Geometry: final body of the model. Coordinates: model frame, mm. A direction names the side the tool comes from. Give positions to 0.01 mm unless a question says otherwise; leave off trailing zeros. Write each loop counter-clockwise with the first axis right and the second up, starting at its lowest first coordinate (ties: lowest second). Pieces come first, ordered by that corner, then holes.
from build123d import *

# Parameters (mm, degrees)
REVOLUTION007_ANGLE     = 180
SKETCH064_W             = 14
SKETCH064_H             = 6
PAD026_DEPTH            = 10
SKETCH063_R             = 1.7
POCKET007_DEPTH         = 38.901
POCKET008_DEPTH         = 28.901
BODY015_PLACEMENT_ANGLE = 75


with BuildPart() as part:
    # Sketch062 → Revolution007 (revolve, symmetric)
    with BuildSketch(Plane.YZ) as revolution007_sk:
        with BuildLine():
            Line((32.9, 0), (32.9, 6.5))
            Line((32.9, 6.5), (29.4, 6.5))
            ThreePointArc((27.9, 8), (28.33934, 6.93934), (29.4, 6.5))
            Line((27.9, 8), (27.9, 11))
            ThreePointArc((29.4, 12.5), (28.33934, 12.06066), (27.9, 11))
            Line((29.4, 12.5), (32.9, 12.5))
            ThreePointArc((38.9, 6.5), (37.142641, 10.742641), (32.9, 12.5))
            Line((38.9, 6.5), (38.9, 0))
            Line((38.9, 0), (38.9, -6.5))
            ThreePointArc((32.9, -12.5), (37.142641, -10.742641), (38.9, -6.5))
            Line((32.9, -12.5), (29.4, -12.5))
            ThreePointArc((27.9, -11), (28.33934, -12.06066), (29.4, -12.5))
            Line((27.9, -11), (27.9, -8))
            ThreePointArc((29.4, -6.5), (28.33934, -6.93934), (27.9, -8))
            Line((29.4, -6.5), (32.9, -6.5))
            Line((32.9, -6.5), (32.9, 0))
        make_face()
    revolve(axis=Axis((0, 0, 0), (0, 0, 1)), revolution_arc=REVOLUTION007_ANGLE / 2)
    revolve(revolution007_sk.sketch, axis=Axis((0, 0, 0), (0, 0, -1)), revolution_arc=REVOLUTION007_ANGLE / 2)

    # Sketch064 (on Face18 of Revolution007) → Pad026 (new body)
    with BuildSketch(Plane(origin=(0, 0, 0), x_dir=(0, 0, -1), z_dir=(0, -1, 0))):
        with Locations((0, 39.4)):
            Rectangle(SKETCH064_W, SKETCH064_H)
        with Locations((0, -39.4)):
            Rectangle(SKETCH064_W, SKETCH064_H)
    extrude(amount=-PAD026_DEPTH)

    # Sketch063 (on Face18 of Revolution007) → Pocket007 (cut, through all)
    with BuildSketch(Plane(origin=(0, 0, 0), x_dir=(0, 0, -1), z_dir=(0, -1, 0))):
        with Locations((4, 39.4)):
            Circle(SKETCH063_R)
        with Locations((-4, 39.4)):
            Circle(SKETCH063_R)
        with Locations((-4, -39.4)):
            Circle(SKETCH063_R)
        with Locations((4, -39.4)):
            Circle(SKETCH063_R)
    extrude(amount=-POCKET007_DEPTH, mode=Mode.SUBTRACT)

    # Sketch065 (on Face22 of Pocket007) → Pocket008 (cut, through all)
    with BuildSketch(Plane.ZX.offset(10)):
        with BuildLine():
            Line((-4, 43.4), (4.000001, 43.4))
            ThreePointArc((4.000001, 35.4), (8, 39.4), (4.000001, 43.4))
            Line((-4, 35.4), (4.000001, 35.4))
            ThreePointArc((-4, 43.4), (-8, 39.4), (-4, 35.4))
        make_face()
        with BuildLine():
            Line((-4, -35.4), (4, -35.4))
            ThreePointArc((4, -43.4), (8, -39.4), (4, -35.4))
            Line((-4, -43.4), (4, -43.4))
            ThreePointArc((-4, -35.4), (-8, -39.4), (-4, -43.4))
        make_face()
    extrude(amount=POCKET008_DEPTH, mode=Mode.SUBTRACT)


with BuildPart() as part_1:
    # Body015 placement: moved
    add(part.part.moved(Location((0, 0, -90.5))).rotate(Axis((0, 0, -90.5), (0, 0, 1)), BODY015_PLACEMENT_ANGLE))


solid = part_1.part
Q1. Access query for faces 1 (the cylindrical face through (-2.67, 37.71, -84.9)), 2 (the flat face through (-15, -38, -97.5)), 3 (the flat face through (6, 40, -97.5)), 4 (the cylindrical face through (-21.17, -31.32, -96.1)), 5 (the cylindrical face through (-14.94, -36.71, -84.8)). Directions: +Z, -Z, +X, -X, +Y, -Y. A direction counts if a zero-diameter tool reaches every point of the face in a straight line with its end or side. Return the directions, or none.
Filled sheet:
face 1: +Y
face 2: -Z, -X, -Y
face 3: -Z, +X, +Y
face 4: -X
face 5: none
Q2. Section A-A on y = 0. Output: boundary loops of the cut face in (x, z), plus the area to 3 significant figures.
Filled sheet:
outline: (-38.9, -97) arc R6 ccw to (-32.9, -103) - (-29.4, -103) arc R1.5 ccw to (-27.9, -101.5) - (-27.9, -98.5) arc R1.5 ccw to (-29.4, -97) - (-32.9, -97) - (-32.9, -84) - (-29.4, -84) arc R1.5 ccw to (-27.9, -82.5) - (-27.9, -79.5) arc R1.5 ccw to (-29.4, -78) - (-32.9, -78) arc R6 ccw to (-38.9, -84) - close
area: 193 mm2
Q3. Pin query (flat end, axial travel): P1, Ø3, axis at x = 6, y = 41, coming from the -Z side; P2, Ø3, axis at x = 7.5, y = 39, coming from the +Z side; P3, Ø4, axis at x = -3, z = -90, coming from the +Y side. Return the tip coordinate at first contact, or that it passes through.
Filled sheet:
P1: stops at z = -97.5
P2: stops at z = -81.22
P3: stops at y = 37.99
Q4. Pull-direction query (Z, two-part tool) for faces 6 (the flat face through (-9.124, -34.05, -90.325)), 7 (the flat face through (-15, -38, -83.5)), 8 (the flat face through (-26, 15, -84)); classes: released by +Z, released by -Z, zero draft, split by the parting line, or undercut.
Filled sheet:
face 6: zero draft
face 7: released by +Z
face 8: undercut
Q5. Section B-B on x = -15.5. Count the separate pieces of the cut face and the enclosed holes in it, plus the area to 3 significant figures.
Filled sheet:
separate pieces: 2
enclosed holes: 2
area: 472 mm2
Q6. Ray query, line 1 along Y through (x, z) = (-11, -94.25); line 2 along Z through (x, y) = (-17, -27.5); line 3 along Y through (x, z) = (-20, -87.5). Return the intervals inside material, ascending.
Filled sheet:
line 1: y = -40.95 to -39.58, -36.1 to -31.01, 31.01 to 37.31
line 2: z = -103 to -97, -84 to -78
line 3: y = -38.54 to -36.85, -31.29 to -26.12, 26.12 to 33.36
